Part model, mm, in its own coordinate system. A direction names the side the tool comes from. Round coordinates to 2 decimals unless told otherwise and drop trailing zeros. Write each loop counter-clockwise with the first axis right and the second up, starting at its lowest first coordinate (ties: lowest second). Pieces come first, ordered by that corner, then holes. Notation, with made-up numbers: M 14.5,-11.5 L 30.5,-11.5 A8 cw 30.5,-6.5 Z; hole C -12,-26.75 d2. An arc over 180 degrees is marked long. Answer as a JSON object with one key per item and string values. Group by question number.
1. Two-plate mould, pull along Z, no slides. Class faces 4 (the face through (95.089, 2, -11)), 5 (the face through (61, 2, -0.74)), 6 (the face through (-23, 2, 11.691)): +Z half, -Z half, draft (parallel to the pull), parting line (faces both ways), or undercut.
2. Drop flat-ended pins along their axis: pin 1 (8.5 mm diameter, centred on x = -4.44, z = 7.41, fed in from -Y); pin 2 (5.5 mm diameter, centred on x = 78.62, z = 7.41, fed in from -Y); pin 3 (1.5 mm diameter, centred on x = 96.5, y = 1.5, fed in from +Z); pin 4 (1.5 mm diameter, centred on x = -22, y = 3, fed in from -Z). Give the stop position or say it passes through.
3. Band-saw the part on B-B, the plane y = 1.65. Write the cut outline in (x, z), plus the area to 3 significant figures.
4. Band-saw the part on D-D, the plane z = 14.75. Write the cut outline in (x, y).
5. Which spindle directions (+Z, -Z, +X, -X, +Y, -Y) get a long thin tool onto all of the face, cutting with end or side? Do faces 1 (the face through (-20.911, 2, 14)), 2 (the face through (40.29, 2.46, -3.96)), 3 (the face through (-23, 2, -8.309)). Say none if no direction does.
6. Band-saw the part on A-A, the plane x = 17. Write the cut outline in (y, z), plus the area to 3 significant figures.
7. Band-saw the part on C-C, the plane z = -4.5. Write the cut outline in (x, y).
8. Drill centre lines: line 1 (Z direction, x = 12.5, y = 2.95); line 2 (X direction, y = 4, z = 6.75); line 3 (Z direction, x = -6.5, y = 1.7). Where is each one in solid material? Low to high. Write a range as from..to.
from build123d import *

# Parameters (mm, degrees)
BOSS_EXTRUDE1_DEPTH = 5


with BuildPart() as part:
    # Sketch2 → Boss-Extrude1 (new body)
    with BuildSketch(Plane(origin=(0, 0, 0), x_dir=(1, 0, 0), z_dir=(0, 1, 0))):
        Polygon((46.589298205, 13.308977097), (51.589298205, 13.308977097), (95.089298205, 13.308977097), (95.089298205, 8.308977097), (100.089298205, 8.308977097), (100.089298205, -11.691022903), (95.089298205, -11.691022903), (95.089298205, -16.691022903), (-20.910701795, -16.691022903), (-20.910701795, -11.691022903), (-25.910701795, -11.691022903), (-25.910701795, 8.308977097), (-20.910701795, 8.308977097), (-20.910701795, 13.308977097), (22.589298205, 13.308977097), (27.589298205, 13.308977097), align=None)
        with BuildLine():
            Line((78.271526231, -10.691022903), (43.271526231, -10.691022903))
            ThreePointArc((43.271526231, -10.691022903), (40.290117596, -7.406437763), (43.271526231, -4.121852623))
            Line((43.271526231, -4.121852623), (78.271526231, -4.121852623))
            ThreePointArc((78.271526231, -4.121852623), (81.920004192, -7.406437763), (78.271526231, -10.691022903))
        make_face(mode=Mode.SUBTRACT)
        with BuildLine():
            Line((-4.092929821, -4.121852623), (30.907070179, -4.121852623))
            ThreePointArc((30.907070179, -4.121852623), (33.888478814, -7.406437763), (30.907070179, -10.691022903))
            Line((30.907070179, -10.691022903), (-4.092929821, -10.691022903))
            ThreePointArc((-4.092929821, -10.691022903), (-7.741407782, -7.406437763), (-4.092929821, -4.121852623))
        make_face(mode=Mode.SUBTRACT)
        with BuildLine():
            Line((-4.092929821, 7.308977097), (30.907070179, 7.308977097))
            ThreePointArc((30.907070179, 7.308977097), (33.888478814, 4.024391957), (30.907070179, 0.739806817))
            Line((30.907070179, 0.739806817), (-4.092929821, 0.739806817))
            ThreePointArc((-4.092929821, 0.739806817), (-7.741407782, 4.024391957), (-4.092929821, 7.308977097))
        make_face(mode=Mode.SUBTRACT)
        with BuildLine():
            Line((78.271526231, 0.739806817), (43.271526231, 0.739806817))
            ThreePointArc((43.271526231, 0.739806817), (40.290117596, 4.024391957), (43.271526231, 7.308977097))
            Line((43.271526231, 7.308977097), (78.271526231, 7.308977097))
            ThreePointArc((78.271526231, 7.308977097), (81.920004192, 4.024391957), (78.271526231, 0.739806817))
        make_face(mode=Mode.SUBTRACT)
    extrude(amount=BOSS_EXTRUDE1_DEPTH)


solid = part.part
Worked answers:
{
 "1": {"face 4": "draft", "face 5": "undercut", "face 6": "+Z half"},
 "2": {"pin 1": "stops at y = 0", "pin 2": "passes through", "pin 3": "stops at z = 11.69", "pin 4": "stops at z = -8.31"},
 "3": {"outline": "M -25.91,-8.31 L -20.91,-8.31 L -20.91,-13.31 L 95.09,-13.31 L 95.09,-8.31 L 100.09,-8.31 L 100.09,11.69 L 95.09,11.69 L 95.09,16.69 L -20.91,16.69 L -20.91,11.69 L -25.91,11.69 Z; hole M -4.09,-7.31 L 30.91,-7.31 A3.3 ccw 30.91,-0.74 L -4.09,-0.74 A3.3 ccw long Z; hole M -4.09,4.12 L 30.91,4.12 A3.3 ccw 30.91,10.69 L -4.09,10.69 A3.3 ccw long Z; hole M 43.27,-7.31 L 78.27,-7.31 A3.3 ccw long 78.27,-0.74 L 43.27,-0.74 A3.3 ccw Z; hole M 43.27,4.12 L 78.27,4.12 A3.3 ccw long 78.27,10.69 L 43.27,10.69 A3.3 ccw Z", "area": "2,620 mm^2"},
 "4": {"outline": "M -20.91,0 L 95.09,0 L 95.09,5 L -20.91,5 Z"},
 "5": {"face 1": "+Z, -X, +Y, -Y", "face 2": "+Y, -Y", "face 3": "-Z, -X, +Y, -Y"},
 "6": {"outline": "M 0,-13.31 L 5,-13.31 L 5,-7.31 L 0,-7.31 Z; M 0,-0.74 L 5,-0.74 L 5,4.12 L 0,4.12 Z; M 0,10.69 L 5,10.69 L 5,16.69 L 0,16.69 Z", "area": "84.3 mm^2"},
 "7": {"outline": "M -25.91,0 L -7.71,0 L -7.71,5 L -25.91,5 Z; M 33.85,0 L 40.32,0 L 40.32,5 L 33.85,5 Z; M 81.89,0 L 100.09,0 L 100.09,5 L 81.89,5 Z"},
 "8": {"line 1": "z = -13.31..-7.31, -0.74..4.12, 10.69..16.69", "line 2": "x = -25.91..-7.68, 33.82..40.36, 81.85..100.09", "line 3": "z = -13.31..-6.6, -1.44..4.83, 9.99..16.69"}
}
